Source: CAD feature listing. Evaluate the final solid. Frame: model axes, mm. Coordinates: 2 decimals unless noted, no trailing zeros. Loops run counter-clockwise (first coordinate to the right, second up) from the corner with the lowest first, then second, coordinate; pieces in that order, holes last.
Item 1: Pin query (flat end, axial travel): pin 1 Ø2 at (x, z) = (1, 49) entering from +Y; pin 2 Ø3 at (x, y) = (-1.5, -20.5) entering from +Z; pin 3 Ø1.3 at (x, y) = (-1.5, 1) entering from +Z. Return the tip coordinate at first contact, or that it passes through.
Item 2: Section query C-C, the plane x = -16.5. Return the cut outline in (y, z) (3 decimals), then the cut area to 3 significant figures.
Item 3: Section query B-B, the plane z = 39.5. Return the cut outline in (x, y) (3 decimals), then the cut area to 3 significant figures.
Item 4: Section query A-A, the plane x = 0. State how many separate pieces and enclosed holes the cut face has, then the cut area to 3 significant figures.
Item 5: Line query: probe 1 along Z at (x, y) = (0, -5); probe 2 along Z at (x, y) = (0, -3.5); probe 3 along Y at (x, z) = (15, 5.5) (3 decimals). Output: solid intervals per line, ascending.
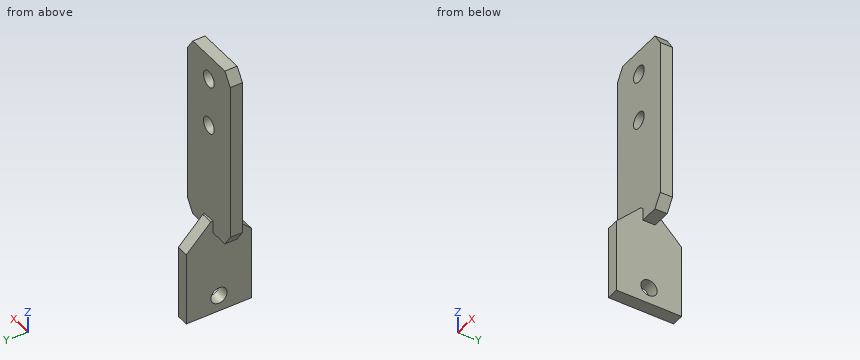
```python
from build123d import *

# Parameters (mm, degrees)
F0_R     = 6.35
F1_DEPTH = 9.525
F3_START = -20.6375
F2_R     = 6.35
F3_DEPTH = 9.525


with BuildPart() as f1:
    # F0 (on Front) → F1 (new body)
    with BuildSketch(Plane.XZ):
        Polygon((-19.05, 147.1890725479), (-25.4, 137.6710385084), (-25.4, 75.7550555281), (-25.4, 13.8390725479), (-19.05, 4.3210385084), (19.05, 4.3210385084), (25.4, 13.8390725479), (25.4, 75.7550555281), (25.4, 137.6710385084), (19.05, 147.1890725479), align=None)
        with Locations((0, 90.0390725479)):
            Circle(F0_R, mode=Mode.SUBTRACT)
        with Locations((0, 128.1390725479)):
            Circle(F0_R, mode=Mode.SUBTRACT)
    extrude(amount=F1_DEPTH)

    # F2 (on face) → F3 (join)
    with BuildSketch(Plane.YZ.offset(25.4).offset(F3_START)):
        Polygon((-9.525, 13.8390725479), (-11.1125, 13.8390725479), (-30.1625, -5.2109274521), (-30.1625, -62.3609274521), (20.6375, -62.3609274521), (20.6375, -5.2109274521), (1.5875, 13.8390725479), (0, 13.8390725479), align=None)
        with Locations((-4.7625, -49.6609274521)):
            Circle(F2_R, mode=Mode.SUBTRACT)
    extrude(amount=-F3_DEPTH)


solid = f1.part
```
Verdict:
1. pin 1: stops at y = 0
1. pin 2: stops at z = 5.95
1. pin 3: stops at z = 13.84
2. outline: (-9.525, 4.321) - (0, 4.321) - (0, 147.189) - (-9.525, 147.189) - close
2. area: 1,360 mm2
3. outline: (-25.4, -9.525) - (25.4, -9.525) - (25.4, 0) - (-25.4, 0) - close
3. area: 484 mm2
4. separate pieces: 3
4. enclosed holes: 1
4. area: 4,410 mm2
5. probe 1: z = -62.36 to -56.01, -43.32 to 83.69, 96.39 to 121.79, 134.49 to 147.19
5. probe 2: z = -62.36 to -55.88, -43.44 to 83.69, 96.39 to 121.79, 134.49 to 147.19
5. probe 3: y = -9.525 to 0
